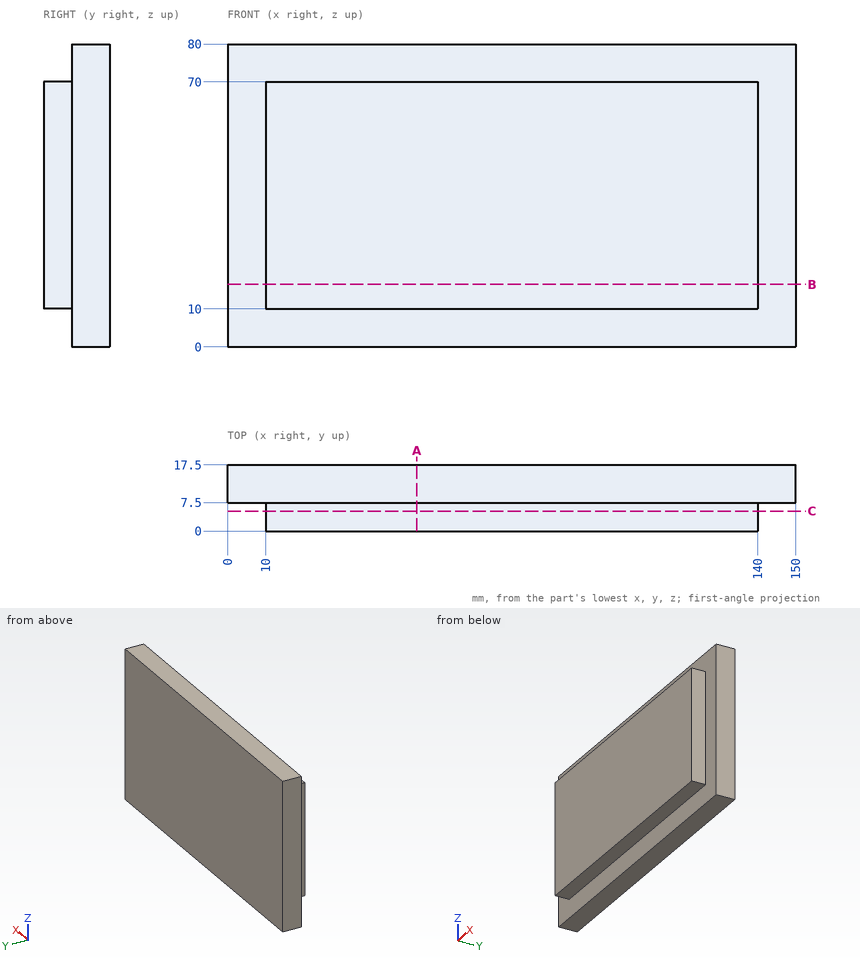
The figure shows three views and two pictorial views of one solid part (mm, origin at its lowest corner). Answer the questions. Give positions to 0.01 mm unless a question says otherwise; leave off trailing zeros. Write each loop counter-clockwise with the first axis right and the second up, starting at its lowest first coordinate (ties: lowest second). Pieces come first, ordered by that corner, then holes. Notation, with made-up numbers: M 49.25,50 L 55.25,50 A27 ccw 55.25,75 Z; hole C 63,-17 d9. An arc over 180 degrees is marked long. One line per item, written item: value. Start each with the question number.
(1) Find the intervals of material crossed by line 1 (X direction, y = 1.5, z = 57); line 2 (Z direction, x = 72, y = 3.25); line 3 (Y direction, x = 17, z = 4.5), in increasing order.
(2) Find section C-C (y = 5.25). Determine the outline of the cut face in (x, z).
(3) Find section B-B (z = 16.5). Determine the outline of the cut face in (x, y).
(4) Find section A-A (x = 50). Determine the outline of the cut face in (y, z), plus the area to 3 significant figures.
(5) Flat-ended cylindrical pins translate along their axes: pin 1 Ø3 at (y, z) = (4, 10) entering from +X; pin 2 Ø2 at (x, y) = (88.5, 3) entering from +Z; pin 3 Ø2 at (y, z) = (5.5, 67.5) entering from -X. Find the tip coordinate at first contact, or state that the pin passes through.
Results below:
1. line 1: x = 10 to 140
1. line 2: z = 10 to 70
1. line 3: y = 7.5 to 17.5
2. outline: M 10,10 L 140,10 L 140,70 L 10,70 Z
3. outline: M 0,7.5 L 10,7.5 L 10,0 L 140,0 L 140,7.5 L 150,7.5 L 150,17.5 L 0,17.5 Z
4. outline: M 0,10 L 7.5,10 L 7.5,0 L 17.5,0 L 17.5,80 L 7.5,80 L 7.5,70 L 0,70 Z
4. area: 1,250 mm^2
5. pin 1: stops at x = 140
5. pin 2: stops at z = 70
5. pin 3: stops at x = 10
